Check sheet for the modelled part. Datum: model origin and axes. Units: mm. Face numbers are marked on the shaded views. A direction names the side the tool comes from. Give positions to 0.01 mm unless a question says otherwise; leave off trailing zeros. Write each loop counter-clockwise with the first axis right and the second up, starting at its lowest first coordinate (ties: lowest second). Pieces come first, ordered by that corner, then holes. Notation, with made-up numbers: (79.5, 27.5) - (118.5, 27.5) arc R35 ccw to (118.5, 66.5) - close; hole circle Ø3 at (-17, 88). An arc over 180 degrees is marked (long way). Return JSON: item names as keys, results as strings. Group by question number.
```python
from build123d import *


with BuildPart() as part:
    # Skizze1 → Rotation1 (revolve)
    with BuildSketch(Plane.XY):
        with BuildLine():
            Line((-2.25, 15), (-2.25, 8.5))
            Line((-2.25, 8.5), (-1.125, 8))
            Line((-1.125, 8), (-1.125, 1.125))
            ThreePointArc((-1.125, 1.125), (-0.795495129, 0.329504871), (0, 0))
            Line((0, 0), (0, 15))
            Line((0, 15), (-2.25, 15))
        make_face()
    revolve(axis=Axis((0, 0, 0), (0, 1, 0)))

    # Skizze2 → Schnitt-Rotation1 (revolve, cut)
    with BuildSketch(Plane.XY):
        Polygon((0, 15), (0, 11), (-1.375, 11), (-1.375, 13), (-1, 13), (-1, 15), align=None)
    revolve(axis=Axis((0, 15, 0), (0, -1, 0)), mode=Mode.SUBTRACT)

    # Skizze3 → Rotation2 (revolve)
    with BuildSketch(Plane.XY):
        with BuildLine():
            Line((-2.25, 12.5), (-2.25, 12))
            ThreePointArc((-2.25, 12), (-2.5, 12.25), (-2.25, 12.5))
        make_face()
        with BuildLine():
            Line((-2.25, 9), (-2.25, 8.5))
            ThreePointArc((-2.25, 8.5), (-2.5, 8.75), (-2.25, 9))
        make_face()
    revolve(axis=Axis((0, 0, 0), (0, 1, 0)))


solid = part.part
```
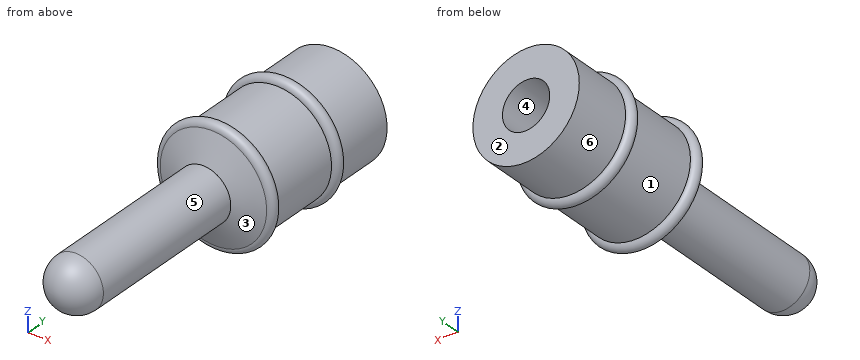
Item 1: Section check C-C on y = 2. Record the cut outline in (x, z) (3 decimals), plus the area to 3 significant figures.
Item 2: Access from +Z, -Z, +X, -X, +Y, -Y to the whole of each face (thin tool, end or side, straight path). Record for the marked faces 5 and 6.
Item 3: Section check A-A on x = 0. Record the cut outline in (y, z) (3 decimals), plus the area to 3 significant figures.
Item 4: Depth check by flat-ended pin: pin 1 (1.8 mm diameter, centred on x = 0, z = 0, fed in from +Y); pin 2 (3 mm diameter, centred on y = 10.5, z = 1, fed in from -X); pin 3 (3 mm diameter, centred on y = 7.5, z = -2, fed in from -X). Enter the tip coordinate at first touch or a pass-through.
Item 5: Section check B-B on z = 0. Record the cut outline in (x, y) (3 decimals), plus the area to 3 significant figures.
Item 6: Material ranges on line 1 along Z through (x, y) = (0, 11.95) (3 decimals); line 2 along Z through (x, y) = (0, 14.2); line 3 along Y through (x, z) = (-0.9, -0.95), recorded low to high. Write a range as from..to.
Item 7: Mould release check, pull along Y, two halves, no side actions. Record for the marked faces 1, 2, 3 and 4: +Y half, -Y half, draft (parallel to the pull), parting line (faces both ways), or undercut.
Reply:
{
 "1": {"outline": "circle Ø2.25 at (0, 0)", "area": "3.98 mm²"},
 "2": {"face 5": "-Y", "face 6": "+Y"},
 "3": {"outline": "(1.125, -1.125) - (8, -1.125) - (8.5, -2.25) arc R0.25 ccw to (9, -2.25) - (12, -2.25) arc R0.25 ccw to (12.5, -2.25) - (15, -2.25) - (15, -1) - (13, -1) - (13, -1.375) - (11, -1.375) - (11, 1.375) - (13, 1.375) - (13, 1) - (15, 1) - (15, 2.25) - (12.5, 2.25) arc R0.25 ccw to (12, 2.25) - (9, 2.25) arc R0.25 ccw to (8.5, 2.25) - (8, 1.125) - (1.125, 1.125) arc R1.125 ccw to start", "area": "39.3 mm²"},
 "4": {"pin 1": "y = 11", "pin 2": "x = -2.25", "pin 3": "x = -2.25"},
 "5": {"outline": "(-2.25, 8.5) - (-1.125, 8) - (-1.125, 1.125) arc R1.125 ccw to (1.125, 1.125) - (1.125, 8) - (2.25, 8.5) arc R0.25 ccw to (2.25, 9) - (2.25, 12) arc R0.25 ccw to (2.25, 12.5) - (2.25, 15) - (1, 15) - (1, 13) - (1.375, 13) - (1.375, 11) - (-1.375, 11) - (-1.375, 13) - (-1, 13) - (-1, 15) - (-2.25, 15) - (-2.25, 12.5) arc R0.25 ccw to (-2.25, 12) - (-2.25, 9) arc R0.25 ccw to start", "area": "39.3 mm²"},
 "6": {"line 1": "-2.25..-1.375, 1.375..2.25", "line 2": "-2.25..-1, 1..2.25", "line 3": "8.08..11, 13..15"},
 "7": {"face 1": "undercut", "face 2": "+Y half", "face 3": "-Y half", "face 4": "draft"}
}
